Drawing for the job (mm, zero at the part's lowest x, y, z). Coordinates: 2 decimals unless noted, no trailing zeros. Write each loop counter-clockwise with the first axis right and the second up, starting at its lowest first coordinate (ties: lowest second). Pieces come first, ordered by that corner, then holes. Notation, with made-up numbers: (47, 70) - (92, 70) arc R21 ccw to (92, 101) - close; hole circle Ø11 at (39, 44). An arc over 180 degrees is marked (long way). Write each question's results on one line, items separated by ' | '.
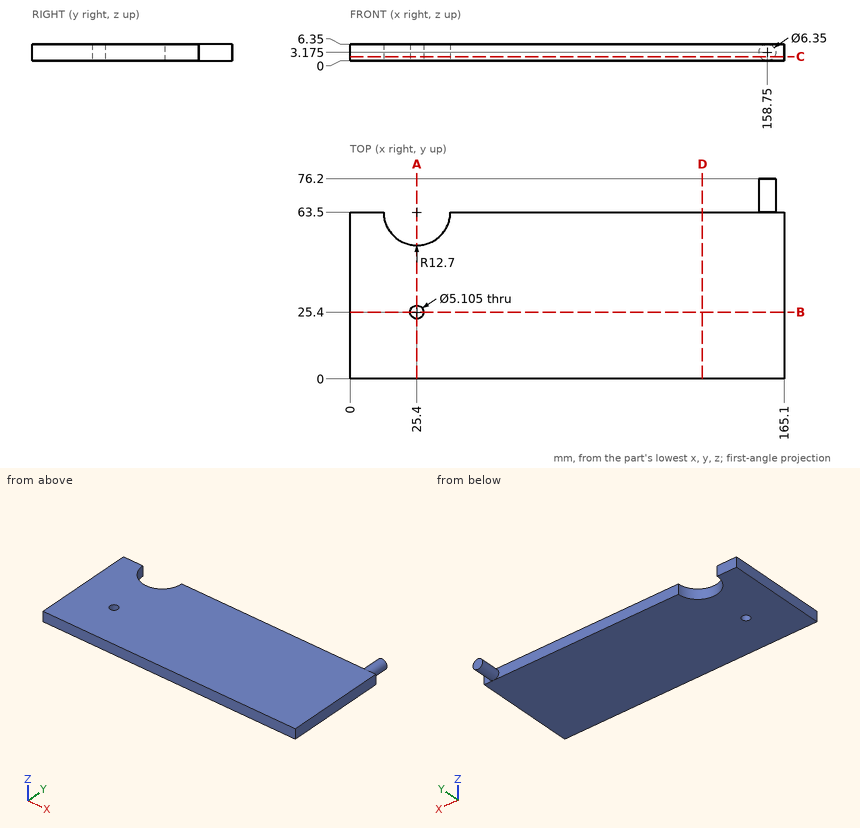
(1) Saw through at A-A on x = 25.4. Write the cut outline in (y, z), then the cut area to 3 significant figures.
Return value:
outline: (0, 0) - (22.85, 0) - (22.85, 6.35) - (0, 6.35) - close; (27.95, 0) - (50.8, 0) - (50.8, 6.35) - (27.95, 6.35) - close | area: 290 mm^2
(2) Saw through at C-C on z = 1.5. Write the cut outline in (x, y) (1 decimal).
Return value:
outline: (0, 0) - (165.1, 0) - (165.1, 63.5) - (161.4, 63.5) - (161.4, 76.2) - (156.1, 76.2) - (156.1, 63.5) - (38.1, 63.5) arc R12.7 cw to (12.7, 63.5) - (0, 63.5) - close; hole circle Ø5.1 at (25.4, 25.4)
(3) Flat gauge pins, fed straight in: P1, Ø3, axis at x = 79.5, z = 3.5, coming from the +Y side; P2, Ø3, axis at x = 25.4, y = 25.4, coming from the +Z side. Where does each tip first touch, or does it go through?
Return value:
P1: stops at y = 63.5 | P2: passes through
(4) Wall check: line 1 (Y direction, x = 25.4, z = 2); line 2 (Y direction, x = 107, z = 6); line 3 (Y direction, x = 17, z = 2.5) (1 decimal). Give the ranges that are in metal, low to high. Write a range as from..to.
Return value:
line 1: y = 0..22.85, 27.95..50.8 | line 2: y = 0..63.5 | line 3: y = 0..54
(5) Saw through at D-D on x = 134. Write the cut outline in (y, z), then the cut area to 3 significant figures.
Return value:
outline: (0, 0) - (63.5, 0) - (63.5, 6.35) - (0, 6.35) - close | area: 403 mm^2
(6) Saw through at B-B on y = 25.4. Write the cut outline in (x, z).
Return value:
outline: (0, 0) - (22.85, 0) - (22.85, 6.35) - (0, 6.35) - close; (27.95, 0) - (165.1, 0) - (165.1, 6.35) - (27.95, 6.35) - close
